Work out the finished part from the listing and answer in its coordinate system (mm). A direction names the side the tool comes from. Coordinates: 2 decimals unless noted, no trailing zeros. Order: outer loops, then holes, each group sorted by start corner. A loop starts at its lowest first (then second) coordinate and runs counter-clockwise, first axis right, second up. Notation, with made-up numbers: (61, 54.5) -> (120, 54.5) arc R16 cw to (120, 65.5) -> close; hole circle Ø4 at (17.25, -6). An arc over 180 degrees is marked (long way). Write item = value, one per line. Start each with the question number.
Q1. The part is cut by section B-B, the plane z = 2.75. Determine the outline of the cut face in (x, y), plus the area to 3 significant figures.
Q2. The part is cut by section D-D, the plane y = -8. Determine the outline of the cut face in (x, z).
Q3. Flat-ended cylindrical pins translate along their axes: pin 1 (4 mm diameter, centred on x = 4.5, z = 0.5, fed in from -Y); pin 2 (4 mm diameter, centred on x = -5.5, z = 7, fed in from +Y); pin 3 (1.5 mm diameter, centred on y = 18, z = -0.5, fed in from +X). Find the tip coordinate at first contact, or state that the pin passes through.
Q4. Which of the six approach directions +Z, -Z, +X, -X, +Y, -Y give full straight-line access (tool end or side, diameter ignored) to faces 1 (the flat face through (-3, 0, 4.318)), 2 (the flat face through (2.5, -2, 0)), 3 (the flat face through (-7.747, -3, 0)), 4 (the flat face through (5, -3.593, 0)), 5 (the cylindrical face through (3.14, 14.61, -0.48))?
Q5. The part is cut by section A-A, the plane y = -3. Determine the outline of the cut face in (x, z), plus the area to 3 significant figures.
Q6. For a pull along X with two mould halves and no side action, classify faces 6 (the cylindrical face through (-5.066, -10.86, 10.116)), 7 (the flat face through (-5, -9.859, 7)), 8 (the cylindrical face through (0.1, 2.5, 0.1)) as +X half, -X half, draft (parallel to the pull), parting line (faces both ways), or undercut.
Q7. The part is cut by section C-C, the plane x = 6. Determine the outline of the cut face in (y, z), plus the area to 3 significant figures.
Q8. Straight lines are drawn through the part: L1, parallel to Z at x = -5.75, y = 2; L2, parallel to X at y = -5, z = 0; L3, parallel to Y at x = 4.5, z = 2. For each, find the intervals that lie inside material, in ascending order. Write a range as from..to.
```python
from build123d import *

# Parameters (mm, degrees)
BOSS_EXTRUDE1_DEPTH = 4.318
CUT_EXTRUDE1_REACH  = 38.412
SKETCH2_W           = 8.541760295
SKETCH2_H           = 11.079108592
SKETCH2_R           = 2.2225
SKETCH3_W           = 5.247
SKETCH3_H           = 2.032
BOSS_EXTRUDE2_DEPTH = 6.35
CUT_EXTRUDE2_DEPTH  = 27.880358119


with BuildPart() as part:
    # Sketch1 → Boss-Extrude1 (new, symmetric)
    with BuildSketch(Plane.XY):
        with BuildLine():
            Line((7.747, -3.592967768), (2.5, -3.592967768))
            Line((2.5, -3.592967768), (2.5, 0))
            ThreePointArc((2.5, 0), (0, 2.5), (-2.5, 0))
            Line((-2.5, 0), (-2.5, -11.890523987))
            Line((-2.5, -11.890523987), (-7.747, -11.890523987))
            Line((-7.747, -11.890523987), (-7.747, 5.76724639))
            Line((-7.747, 5.76724639), (2.873732949, 5.611740799))
            Line((2.873732949, 5.611740799), (2.873732949, 23.425016961))
            Line((2.873732949, 23.425016961), (7.747, 23.425016961))
            Line((7.747, 23.425016961), (7.747, -3.592967768))
        make_face()
    extrude(amount=BOSS_EXTRUDE1_DEPTH, both=True)

    # Cut-Extrude1: up to this plane
    cut_extrude1_end = Plane(origin=(2.873732949, 5.611740799, 4.318), z_dir=(-0.014640131281330963, -0.9998928275350643, 0))
    # Sketch2 → Cut-Extrude1 (cut, up to the surface)
    with BuildSketch(Plane(origin=(0, 23.425016961, 0), x_dir=(1, 0, 0), z_dir=(0, 1, 0)), mode=Mode.PRIVATE) as cut_extrude1_sk1:
        with Locations((5.587976973, 0.096845355)):
            Rectangle(SKETCH2_W, SKETCH2_H)
        with Locations(Location((5.310366443, 0, 0), (0, 0, 270))):
            Circle(SKETCH2_R, mode=Mode.SUBTRACT)
    cut_extrude1_tool1 = split(extrude(cut_extrude1_sk1.sketch, amount=-CUT_EXTRUDE1_REACH, mode=Mode.PRIVATE), bisect_by=cut_extrude1_end, keep=Keep.BOTH, mode=Mode.PRIVATE)
    add(cut_extrude1_tool1.solids().sort_by_distance((5.587977, 23.425017, -5.496504))[0], mode=Mode.SUBTRACT)

    # Sketch3 → Boss-Extrude2 (add)
    with BuildSketch(Plane.XY.offset(4.318)):
        with Locations((-5.1235, -10.874523987)):
            Rectangle(SKETCH3_W, SKETCH3_H)
    extrude(amount=BOSS_EXTRUDE2_DEPTH)

    # Sketch4 → Cut-Extrude2 (cut, through all)
    with BuildSketch(Plane(origin=(0, 0, 0), x_dir=(1, 0, 0), z_dir=(0, 1, 0))):
        with BuildLine():
            Line((-7.747, -7.493), (-9.552186856, -7.493))
            Line((-9.552186856, -7.493), (-9.552186856, -11.539215141))
            Line((-9.552186856, -11.539215141), (-1.066763887, -11.539215141))
            Line((-1.066763887, -11.539215141), (-1.066763887, -7.493))
            Line((-1.066763887, -7.493), (-2.5, -7.493))
            ThreePointArc((-2.5, -7.493), (-5.1235, -10.1165), (-7.747, -7.493))
        make_face()
    extrude(amount=-CUT_EXTRUDE2_DEPTH, mode=Mode.SUBTRACT)


solid = part.part
```
Model answer:
q1.outline = (-7.75, -11.89) -> (-2.5, -11.89) -> (-2.5, 0) arc R2.5 cw to (2.5, 0) -> (2.5, -3.59) -> (7.75, -3.59) -> (7.75, 5.54) -> (-7.75, 5.77) -> close
q1.area = 159 mm2
q2.outline = (-7.75, -4.32) -> (-2.5, -4.32) -> (-2.5, 4.32) -> (-7.75, 4.32) -> close
q3.pin_1 = -3.59
q3.pin_2 = -9.86
q3.pin_3 = 7.53
q4.face_1 = +Z, +X, -X, +Y
q4.face_2 = +Z, -Z, -Y
q4.face_3 = +Z, -Z, -X, +Y, -Y
q4.face_4 = +Z, -Z, +X, -Y
q4.face_5 = +Y
q5.outline = (-7.75, -4.32) -> (-2.5, -4.32) -> (-2.5, 4.32) -> (-7.75, 4.32) -> close; (2.5, -4.32) -> (7.75, -4.32) -> (7.75, 4.32) -> (2.5, 4.32) -> close
q5.area = 90.6 mm2
q6.face_6 = parting line
q6.face_7 = draft
q6.face_8 = undercut
q7.outline = (-3.59, -4.32) -> (5.57, -4.32) -> (5.57, -2.11) -> (23.43, -2.11) -> (23.43, 2.11) -> (5.57, 2.11) -> (5.57, 4.32) -> (-3.59, 4.32) -> close
q7.area = 155 mm2
q8.L1 = -4.32..4.32
q8.L2 = -7.75..-2.5
q8.L3 = -3.59..23.43
